Input: part model. Units: mm. Frame: model coordinates. Face numbers are marked on the shaded views. A direction names the side the tool comes from. Give positions to 0.01 mm unless a question says otherwise; leave off trailing zeros. Write each loop counter-clockwise with the first axis right and the second up, starting at its lowest first coordinate (ties: lowest second). Pieces come first, ordered by that corner, then holes. Notation, with made-up numbers: (62.25, -30.5) - (78.25, -30.5) arc R10 cw to (78.25, -24.5) - close; hole circle Ø2 at (-13.75, 43.25). An arc over 180 degrees is marked (long way). Use a Markdown table: item, result. Add a question column.
1. Material intervals for probe 1 along Y at (x, z) = (-2, 23.5); probe 2 along Z at (x, y) = (11.5, 261); probe 3 along X at (y, z) = (253, 14), sorted ascending.
2. Pin query (flat end, axial travel): pin 1 (4 mm diameter, centred on x = 4.5, z = 6, fed in from +Y); pin 2 (3 mm diameter, centred on x = 19, z = 40, fed in from -Y); pin 3 (10 mm diameter, centred on x = -18, z = 11, fed in from -Y); pin 4 (6 mm diameter, centred on y = -15, z = 40, fed in from -X). Return the tip coordinate at first contact, or that it passes through.
3. Section query B-B, the plane y = 8. Return loops of the section in (x, z), plus the area to 3 significant figures.
4. Section query A-A, the plane y = 214. Return loops of the section in (x, z), plus the area to 3 significant figures.
5. Set-up query: the marked faces 1, 2, 3, 4 and 5. Return all of +Z, -Z, +X, -X, +Y, -Y with unobstructed straight access to the full face (end or side cutting, diameter ignored); none if empty.
6. Mould query, pull axis Y, two halves, no side actions, for the marked faces 6, 7 and 8. Classes: released by +Y, released by -Y, zero draft, split by the parting line, or undercut.
```python
from build123d import *

# Parameters (mm, degrees)
BOSS_EXTRUDE1_DEPTH = 50
CUT_EXTRUDE4_DEPTH  = 10
CUT_EXTRUDE5_DEPTH  = 10
SKETCH6_R           = 15
CUT_EXTRUDE6_DEPTH  = 301.947465254
CUT_EXTRUDE7_DEPTH  = 301.947465254
SKETCH8_W           = 30
SKETCH8_H           = 5
CUT_EXTRUDE8_DEPTH  = 346.907627132
SKETCH9_W           = 40
SKETCH9_H           = 50
BOSS_EXTRUDE2_DEPTH = 30
FILLET1_R           = 10
SKETCH10_W          = 30
SKETCH10_H          = 25
CUT_EXTRUDE9_DEPTH  = 347.377087182
SKETCH11_R          = 5
CUT_EXTRUDE10_DEPTH = 347.917982419


with BuildPart() as part:
    # Sketch1 → Boss-Extrude1 (new body)
    with BuildSketch(Plane.XY):
        Polygon((0, 0), (30, 0), (30, 300), (1.321178182, 340.957602214), (-28.678821818, 319.951376068), (0, 278.993773854), align=None)
    extrude(amount=BOSS_EXTRUDE1_DEPTH)

    # Sketch3 → Cut-Extrude4 (cut)
    with BuildSketch(Plane.XY.offset(50)):
        Polygon((30, 300), (0, 278.993773854), (0, 5), (30, 5), align=None)
    extrude(amount=-CUT_EXTRUDE4_DEPTH, mode=Mode.SUBTRACT)

    # Sketch4 → Cut-Extrude5 (cut)
    with BuildSketch(Plane(origin=(0, 0, 0), x_dir=(-1, 0, 0), z_dir=(0, 0, -1))):
        Polygon((-30, 300), (0, 278.993773854), (0, 5), (-30, 5), align=None)
    extrude(amount=-CUT_EXTRUDE5_DEPTH, mode=Mode.SUBTRACT)

    # Sketch6 → Cut-Extrude6 (cut, through all)
    with BuildSketch(Plane(origin=(161.084195268, 112.792367813, 0), x_dir=(0, 0, -1), z_dir=(0.819152044288991, 0.5735764363510472, 0))):
        with Locations(Location((-25, 253.538320196, 0), (0, 0, 90))):
            Circle(SKETCH6_R)
    extrude(amount=-CUT_EXTRUDE6_DEPTH, mode=Mode.SUBTRACT)

    # Sketch7 → Cut-Extrude7 (cut, through all)
    with BuildSketch(Plane(origin=(161.084195268, 112.792367813, 0), x_dir=(0, 0, -1), z_dir=(0.819152044288991, 0.5735764363510472, 0))):
        with BuildLine():
            Line((-50, 228.538320196), (-40, 228.538320196))
            Line((-40, 228.538320196), (-40, 233.538320196))
            ThreePointArc((-40, 233.538320196), (-47.360679775, 242.357980309), (-50, 253.538320196))
            Line((-50, 253.538320196), (-50, 228.538320196))
        make_face()
        with BuildLine():
            Line((-50, 278.538320196), (-50, 253.538320196))
            ThreePointArc((-50, 253.538320196), (-42.67766953, 271.215989726), (-25, 278.538320196))
            Line((-25, 278.538320196), (-50, 278.538320196))
        make_face()
        with BuildLine():
            Line((0, 278.538320196), (-25, 278.538320196))
            ThreePointArc((-25, 278.538320196), (-7.32233047, 271.215989726), (0, 253.538320196))
            Line((0, 253.538320196), (0, 278.538320196))
        make_face()
        with BuildLine():
            Line((0, 228.538320196), (0, 253.538320196))
            ThreePointArc((0, 253.538320196), (-2.639320225, 242.357980309), (-10, 233.538320196))
            Line((-10, 233.538320196), (-10, 228.538320196))
            Line((-10, 228.538320196), (0, 228.538320196))
        make_face()
    extrude(amount=-CUT_EXTRUDE7_DEPTH, mode=Mode.SUBTRACT)

    # Sketch8 → Cut-Extrude8 (cut, through all)
    with BuildSketch(Plane.XY.offset(50)):
        with Locations((15, 2.5)):
            Rectangle(SKETCH8_W, SKETCH8_H)
    extrude(amount=-CUT_EXTRUDE8_DEPTH, mode=Mode.SUBTRACT)

    # Sketch9 → Boss-Extrude2 (add)
    with BuildSketch(Plane.XZ.offset(-5)):
        with Locations((15, 25)):
            Rectangle(SKETCH9_W, SKETCH9_H)
    extrude(amount=BOSS_EXTRUDE2_DEPTH)

    # Fillet1
    # the kernel refuses this fillet: 10 mm, written as the material it adds along each edge
    with BuildSketch(Plane(origin=(0, 5, 40), x_dir=(-1, 0, 0), z_dir=(0, 0, -1))) as fillet1_piece_1:
        with BuildLine():
            CenterArc((10, 8.660254038), FILLET1_R, 180, 60)
            Line((0, 8.660254038), (0, 0))
            Line((0, 0), (5, 0))
        make_face()
    extrude(amount=30)
    with BuildSketch(Plane(origin=(30, 5, 40), x_dir=(1, 0, 0), z_dir=(0, 0, -1))) as fillet1_piece_2:
        with BuildLine():
            CenterArc((10, -8.660254038), FILLET1_R, 120, 60)
            Line((0, -8.660254038), (0, 0))
            Line((0, 0), (5, 0))
        make_face()
    extrude(amount=30)
    with BuildSketch(Plane(origin=(0, 5, 40), x_dir=(0, 0, 1), z_dir=(1, 0, 0))) as fillet1_piece_3:
        with BuildLine():
            CenterArc((FILLET1_R, -FILLET1_R), FILLET1_R, 90, 90)
            Line((0, -FILLET1_R), (0, 0))
            Line((0, 0), (FILLET1_R, 0))
        make_face()
    extrude(amount=30)
    with BuildSketch(Plane(origin=(0, 5, 10), x_dir=(0, 0, -1), z_dir=(1, 0, 0))) as fillet1_piece_4:
        with BuildLine():
            CenterArc((FILLET1_R, FILLET1_R), FILLET1_R, 180, 90)
            Line((0, FILLET1_R), (0, 0))
            Line((0, 0), (FILLET1_R, 0))
        make_face()
    extrude(amount=30)
    with BuildSketch(Plane(origin=(-25, 5, 40), x_dir=(0, 0, 1), z_dir=(1, 0, 0))) as fillet1_piece_5a_section:
        with BuildLine():
            CenterArc((FILLET1_R, -FILLET1_R), FILLET1_R, 90, 90)
            Line((0, -FILLET1_R), (0, 0))
            Line((0, 0), (FILLET1_R, 0))
        make_face()
    fillet1_piece_5a = extrude(amount=55, mode=Mode.PRIVATE)
    fillet1_piece_5a = split(fillet1_piece_5a, bisect_by=Plane(origin=(-5, 5, 40), z_dir=(1, 0, 0)), keep=Keep.TOP, mode=Mode.PRIVATE)
    fillet1_piece_5a = split(fillet1_piece_5a, bisect_by=Plane(origin=(0, 5, 40), z_dir=(-1, 0, 0)), keep=Keep.TOP, mode=Mode.PRIVATE)
    with BuildSketch(Plane(origin=(0, 5, 61.650635095), x_dir=(-1, 0, 0), z_dir=(0, 0, -1))) as fillet1_piece_5b_section:
        with BuildLine():
            CenterArc((10, 8.660254038), FILLET1_R, 180, 60)
            Line((0, 8.660254038), (0, 0))
            Line((0, 0), (5, 0))
        make_face()
    fillet1_piece_5b = extrude(amount=51.650635095, mode=Mode.PRIVATE)
    fillet1_piece_5b = split(fillet1_piece_5b, bisect_by=Plane(origin=(0, 5, 50), z_dir=(0, 0, -1)), keep=Keep.TOP, mode=Mode.PRIVATE)
    fillet1_piece_5b = split(fillet1_piece_5b, bisect_by=Plane(origin=(0, 5, 40), z_dir=(0, 0, 1)), keep=Keep.TOP, mode=Mode.PRIVATE)
    fillet1_piece_5 = fillet1_piece_5a & fillet1_piece_5b
    add(fillet1_piece_5)
    with BuildSketch(Plane(origin=(-25, 5, 10), x_dir=(0, 0, -1), z_dir=(1, 0, 0))) as fillet1_piece_6a_section:
        with BuildLine():
            CenterArc((FILLET1_R, FILLET1_R), FILLET1_R, 180, 90)
            Line((0, FILLET1_R), (0, 0))
            Line((0, 0), (FILLET1_R, 0))
        make_face()
    fillet1_piece_6a = extrude(amount=55, mode=Mode.PRIVATE)
    fillet1_piece_6a = split(fillet1_piece_6a, bisect_by=Plane(origin=(-5, 5, 10), z_dir=(1, 0, 0)), keep=Keep.TOP, mode=Mode.PRIVATE)
    fillet1_piece_6a = split(fillet1_piece_6a, bisect_by=Plane(origin=(0, 5, 10), z_dir=(-1, 0, 0)), keep=Keep.TOP, mode=Mode.PRIVATE)
    with BuildSketch(Plane(origin=(0, 5, 40), x_dir=(-1, 0, 0), z_dir=(0, 0, -1))) as fillet1_piece_6b_section:
        with BuildLine():
            CenterArc((10, 8.660254038), FILLET1_R, 180, 60)
            Line((0, 8.660254038), (0, 0))
            Line((0, 0), (5, 0))
        make_face()
    fillet1_piece_6b = extrude(amount=51.650635095, mode=Mode.PRIVATE)
    fillet1_piece_6b = split(fillet1_piece_6b, bisect_by=Plane(origin=(0, 5, 0), z_dir=(0, 0, 1)), keep=Keep.TOP, mode=Mode.PRIVATE)
    fillet1_piece_6b = split(fillet1_piece_6b, bisect_by=Plane(origin=(0, 5, 10), z_dir=(0, 0, -1)), keep=Keep.TOP, mode=Mode.PRIVATE)
    fillet1_piece_6 = fillet1_piece_6a & fillet1_piece_6b
    add(fillet1_piece_6)
    with BuildSketch(Plane(origin=(0, 5, 40), x_dir=(0, 0, 1), z_dir=(1, 0, 0))) as fillet1_piece_7a_section:
        with BuildLine():
            CenterArc((FILLET1_R, -FILLET1_R), FILLET1_R, 90, 90)
            Line((0, -FILLET1_R), (0, 0))
            Line((0, 0), (FILLET1_R, 0))
        make_face()
    fillet1_piece_7a = extrude(amount=55, mode=Mode.PRIVATE)
    fillet1_piece_7a = split(fillet1_piece_7a, bisect_by=Plane(origin=(35, 5, 40), z_dir=(-1, 0, 0)), keep=Keep.TOP, mode=Mode.PRIVATE)
    fillet1_piece_7a = split(fillet1_piece_7a, bisect_by=Plane(origin=(30, 5, 40), z_dir=(1, 0, 0)), keep=Keep.TOP, mode=Mode.PRIVATE)
    with BuildSketch(Plane(origin=(30, 5, 61.650635095), x_dir=(1, 0, 0), z_dir=(0, 0, -1))) as fillet1_piece_7b_section:
        with BuildLine():
            CenterArc((10, -8.660254038), FILLET1_R, 120, 60)
            Line((0, -8.660254038), (0, 0))
            Line((0, 0), (5, 0))
        make_face()
    fillet1_piece_7b = extrude(amount=51.650635095, mode=Mode.PRIVATE)
    fillet1_piece_7b = split(fillet1_piece_7b, bisect_by=Plane(origin=(30, 5, 50), z_dir=(0, 0, -1)), keep=Keep.TOP, mode=Mode.PRIVATE)
    fillet1_piece_7b = split(fillet1_piece_7b, bisect_by=Plane(origin=(30, 5, 40), z_dir=(0, 0, 1)), keep=Keep.TOP, mode=Mode.PRIVATE)
    fillet1_piece_7 = fillet1_piece_7a & fillet1_piece_7b
    add(fillet1_piece_7)
    with BuildSketch(Plane(origin=(30, 5, 40), x_dir=(1, 0, 0), z_dir=(0, 0, -1))) as fillet1_piece_8a_section:
        with BuildLine():
            CenterArc((10, -8.660254038), FILLET1_R, 120, 60)
            Line((0, -8.660254038), (0, 0))
            Line((0, 0), (5, 0))
        make_face()
    fillet1_piece_8a = extrude(amount=51.650635095, mode=Mode.PRIVATE)
    fillet1_piece_8a = split(fillet1_piece_8a, bisect_by=Plane(origin=(30, 5, 0), z_dir=(0, 0, 1)), keep=Keep.TOP, mode=Mode.PRIVATE)
    fillet1_piece_8a = split(fillet1_piece_8a, bisect_by=Plane(origin=(30, 5, 10), z_dir=(0, 0, -1)), keep=Keep.TOP, mode=Mode.PRIVATE)
    with BuildSketch(Plane(origin=(0, 5, 10), x_dir=(0, 0, -1), z_dir=(1, 0, 0))) as fillet1_piece_8b_section:
        with BuildLine():
            CenterArc((FILLET1_R, FILLET1_R), FILLET1_R, 180, 90)
            Line((0, FILLET1_R), (0, 0))
            Line((0, 0), (FILLET1_R, 0))
        make_face()
    fillet1_piece_8b = extrude(amount=55, mode=Mode.PRIVATE)
    fillet1_piece_8b = split(fillet1_piece_8b, bisect_by=Plane(origin=(35, 5, 10), z_dir=(-1, 0, 0)), keep=Keep.TOP, mode=Mode.PRIVATE)
    fillet1_piece_8b = split(fillet1_piece_8b, bisect_by=Plane(origin=(30, 5, 10), z_dir=(1, 0, 0)), keep=Keep.TOP, mode=Mode.PRIVATE)
    fillet1_piece_8 = fillet1_piece_8a & fillet1_piece_8b
    add(fillet1_piece_8)
    # the kernel refuses this fillet: 10 mm, written as the material it takes off along each edge
    with BuildSketch(Plane(origin=(60, -25, 0), x_dir=(0, 1, 0), z_dir=(-1, 0, 0)), Plane(origin=(-30, -25, 50), x_dir=(0, 1, 0), z_dir=(1, 0, 0))) as fillet1_2_piece_1:
        with BuildLine():
            CenterArc((FILLET1_R, -FILLET1_R), FILLET1_R, 90, 90)
            Line((0, -FILLET1_R), (0, 0))
            Line((0, 0), (FILLET1_R, 0))
        make_face()
    extrude(amount=90, mode=Mode.SUBTRACT)

    # Sketch10 → Cut-Extrude9 (cut, through all)
    with BuildSketch(Plane(origin=(0, 0, 0), x_dir=(-1, 0, 0), z_dir=(0, 0, -1))):
        with Locations((-15, -12.5)):
            Rectangle(SKETCH10_W, SKETCH10_H)
    extrude(amount=-CUT_EXTRUDE9_DEPTH, mode=Mode.SUBTRACT)

    # Sketch11 → Cut-Extrude10 (cut, through all)
    with BuildSketch(Plane.ZY.offset(5)):
        with Locations((10, -15)):
            Circle(SKETCH11_R)
        with Locations((40, -15)):
            Circle(SKETCH11_R)
    extrude(amount=-CUT_EXTRUDE10_DEPTH, mode=Mode.SUBTRACT)


solid = part.part
```
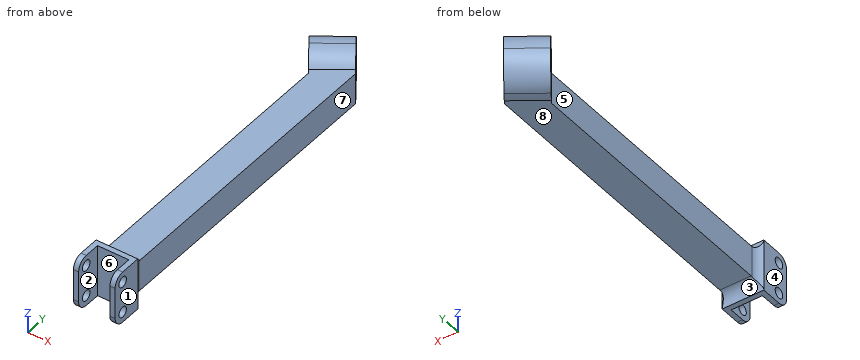
Result sheet:
| question | item | result |
|---|---|---|
| 1 | probe 1 | y = -25 to 7.66, 281.85 to 289.89, 326.33 to 338.58 |
| 1 | probe 2 | z = 10 to 40 |
| 1 | probe 3 | x = 0 to 30 |
| 2 | pin 1 | stops at y = 335.39 |
| 2 | pin 2 | stops at y = 0 |
| 2 | pin 3 | stops at y = 297.66 |
| 2 | pin 4 | passes through |
| 3 | outline | (-1.76, 7.14) - (31.76, 7.14) - (31.76, 42.86) - (-1.76, 42.86) - close |
| 3 | area | 1,200 mm² |
| 4 | outline | (0, 10) - (30, 10) - (30, 40) - (0, 40) - close |
| 4 | area | 900 mm² |
| 5 | face 1 | +Z, -Z, +X, +Y, -Y |
| 5 | face 2 | +Z, -Z, -Y |
| 5 | face 3 | -Z, +X, -X |
| 5 | face 4 | +Z, -Z, -X, -Y |
| 5 | face 5 | +Z, -Z, -X |
| 6 | face 6 | released by -Y |
| 6 | face 7 | zero draft |
| 6 | face 8 | undercut |
